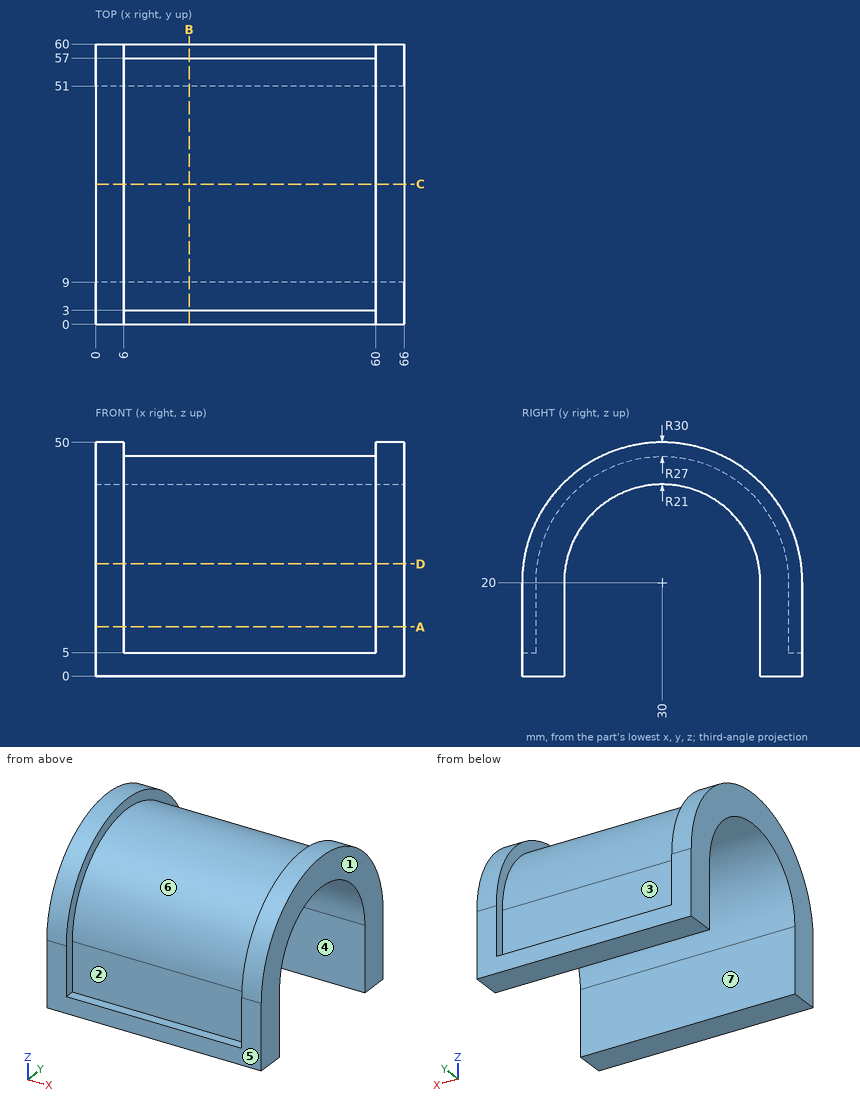
Check sheet for the drawn part. Datum: minimum x, y, z corner. Units: mm. A direction names the side the tool comes from. Coordinates: 2 decimals unless noted, no trailing zeros. Loops run counter-clockwise (first coordinate to the right, second up) from the corner with the lowest first, then second, coordinate; pieces in that order, holes last. Notation, with made-up numbers: M 75,-28 L 106,-28 A28 ccw 106,11 Z; hole C 11,-32 d7. An arc over 180 degrees is marked long. Answer as a JSON object with one key per item and string values.
1. Scan lines: L1, parallel to Y at x = 14.5, z = 8; L2, parallel to Y at x = 29.5, z = 4.5; L3, parallel to X at y = 54.5, z = 31.5. Record each from-to range of solid material in increasing order. Write a range as from..to.
Outcome:
{"L1": "3..9, 51..57", "L2": "0..9, 51..60", "L3": "0..6, 60..66"}
2. Release check for a two-part mould opening along Y. For the marked faces 4, 5, 6 and 7 record: pulls with the +Y half, pulls with the -Y half, needs draft (parallel to the pull), parting line crosses it, or undercut.
Outcome:
{"face 4": "undercut", "face 5": "pulls with the -Y half", "face 6": "parting line crosses it", "face 7": "undercut"}
3. Sectioned sample at A-A on z = 10.5. Record the cut outline in (x, y).
Outcome:
{"outline": "M 0,0 L 6,0 L 6,3 L 60,3 L 60,0 L 66,0 L 66,9 L 0,9 Z; M 0,51 L 66,51 L 66,60 L 60,60 L 60,57 L 6,57 L 6,60 L 0,60 Z"}
4. Access from +Z, -Z, +X, -X, +Y, -Y to the whole of each face (thin tool, end or side, straight path). Record for the marked faces 1, 2 and 3.
Outcome:
{"face 1": "+Z, -Z, +X, +Y, -Y", "face 2": "+Z, -Y", "face 3": "+Z, +Y"}
5. Depth check by flat-ended pin: P1, Ø3, axis at x = 16, y = 35.5, coming from the -Z side; P2, Ø1.5, axis at x = 44.5, y = 14, coming from the -Z side; P3, Ø1, axis at x = 17.5, z = 15, coming from the +Y side. Enter the tip coordinate at first touch or a pass-through.
Outcome:
{"P1": "z = 39.8", "P2": "z = 32.67", "P3": "y = 57"}
6. Sectioned sample at C-C on y = 30. Record the cut outline in (x, z).
Outcome:
{"outline": "M 0,41 L 66,41 L 66,50 L 60,50 L 60,47 L 6,47 L 6,50 L 0,50 Z"}
7. Sectioned sample at D-D on z = 24. Record the cut outline in (x, y).
Outcome:
{"outline": "M 0,0.27 L 6,0.27 L 6,3.3 L 60,3.3 L 60,0.27 L 66,0.27 L 66,9.38 L 0,9.38 Z; M 0,50.62 L 66,50.62 L 66,59.73 L 60,59.73 L 60,56.7 L 6,56.7 L 6,59.73 L 0,59.73 Z"}
8. Sectioned sample at B-B on x = 20. Record the cut outline in (y, z), and give its area (3 significant figures).
Outcome:
{"outline": "M 0,0 L 9,0 L 9,20 A21 cw 51,20 L 51,0 L 60,0 L 60,5 L 57,5 L 57,20 A27 ccw 3,20 L 3,5 L 0,5 Z", "area": "722 mm²"}
